from build123d import *

# Parameters (mm, degrees)
SKETCH1_R           = 2.5
BOSS_EXTRUDE1_DEPTH = 0.8


with BuildPart() as part:
    # Sketch1 → Boss-Extrude1 (new body)
    with BuildSketch(Plane(origin=(0, 0, 0), x_dir=(1, 0, 0), z_dir=(0, 1, 0))):
        with BuildLine():
            Line((5, 0), (208.1, 0))
            ThreePointArc((208.1, 0), (211.635533906, -1.464466094), (213.1, -5))
            Line((213.1, -5), (213.1, -82.7))
            Line((213.1, -82.7), (213.1, -87.7))
            Line((213.1, -87.7), (213.1, -89.7))
            ThreePointArc((213.1, -89.7), (212.221320344, -91.821320344), (210.1, -92.7))
            Line((210.1, -92.7), (196.1, -92.7))
            ThreePointArc((196.1, -92.7), (193.978679656, -93.578679656), (193.1, -95.7))
            Line((193.1, -95.7), (193.1, -102.7))
            Line((193.1, -102.7), (193.1, -107.7))
            Line((193.1, -107.7), (188.1, -107.7))
            Line((188.1, -107.7), (5, -107.7))
            ThreePointArc((5, -107.7), (1.464466094, -106.235533906), (0, -102.7))
            Line((0, -102.7), (0, -5))
            ThreePointArc((0, -5), (1.464466094, -1.464466094), (5, 0))
        make_face()
        with Locations((73.6, -22.2)):
            Circle(SKETCH1_R, mode=Mode.SUBTRACT)
        with Locations((115.6, -22.2)):
            Circle(SKETCH1_R, mode=Mode.SUBTRACT)
        with Locations((115.6, -64.2)):
            Circle(SKETCH1_R, mode=Mode.SUBTRACT)
        with Locations((73.6, -64.2)):
            Circle(SKETCH1_R, mode=Mode.SUBTRACT)
    extrude(amount=BOSS_EXTRUDE1_DEPTH)


solid = part.part
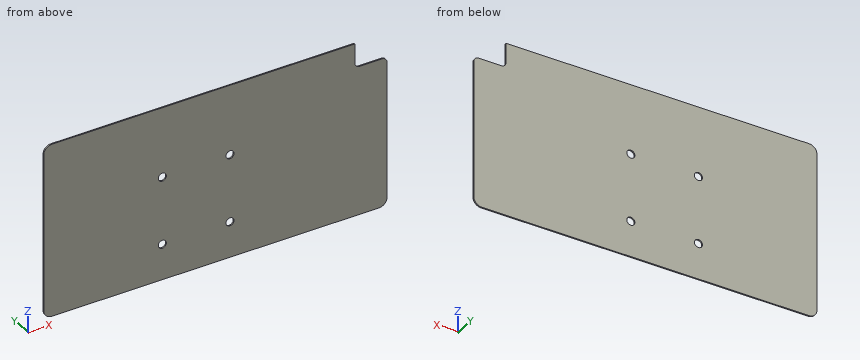
Source: CAD feature listing. Evaluate the final solid. Frame: model axes, mm. Coordinates: 2 decimals unless noted, no trailing zeros. Loops run counter-clockwise (first coordinate to the right, second up) from the corner with the lowest first, then second, coordinate; pieces in that order, holes last. Notation, with made-up numbers: M -13.5,68 L 40.5,68 A32 ccw 40.5,103 Z; hole C 43.25,-30.5 d9. An arc over 180 degrees is marked long. Answer in a Markdown table with one row per item.
Q1. Section A-A on z = 64.2. Return the cut outline in (x, y).
Answers below:
| item | result |
|---|---|
| outline | M 0,0 L 71.1,0 L 71.1,0.8 L 0,0.8 Z; M 76.1,0 L 113.1,0 L 113.1,0.8 L 76.1,0.8 Z; M 118.1,0 L 213.1,0 L 213.1,0.8 L 118.1,0.8 Z |
Q2. Ray query, probe 1 along X at (y, z) = (0.25, 22.2); probe 2 along Z at (x, y) = (115.6, 0.6); probe 3 along Z at (x, y) = (197, 0.7). Return the intervals inside material, ascending. Write a range as from..to.
Answers below:
| item | result |
|---|---|
| probe 1 | x = 0..71.1, 76.1..113.1, 118.1..213.1 |
| probe 2 | z = 0..19.7, 24.7..61.7, 66.7..107.7 |
| probe 3 | z = 0..92.7 |
Q3. Section B-B on x = 115.6. Return the cut outline in (y, z), plus the area to 3 significant figures.
Answers below:
| item | result |
|---|---|
| outline | M 0,0 L 0.8,0 L 0.8,19.7 L 0,19.7 Z; M 0,24.7 L 0.8,24.7 L 0.8,61.7 L 0,61.7 Z; M 0,66.7 L 0.8,66.7 L 0.8,107.7 L 0,107.7 Z |
| area | 78.2 mm^2 |
Q4. Section C-C on y = 0.55. Return the cut outline in (x, z), plus the area to 3 significant figures.
Answers below:
| item | result |
|---|---|
| outline | M 0,5 A5 ccw 5,0 L 208.1,0 A5 ccw 213.1,5 L 213.1,89.7 A3 ccw 210.1,92.7 L 196.1,92.7 A3 cw 193.1,95.7 L 193.1,107.7 L 5,107.7 A5 ccw 0,102.7 Z; hole C 73.6,22.2 d5; hole C 73.6,64.2 d5; hole C 115.6,22.2 d5; hole C 115.6,64.2 d5 |
| area | 22,600 mm^2 |
